Input: dimensioned drawing with shaded views. Units: mm. Origin: part minimum x, y, z. Give positions to 0.01 mm unless a question says otherwise; leave off trailing zeros. Write each loop counter-clockwise with the first axis right and the second up, starting at its lowest first coordinate (ties: lowest second). Pieces come first, ordered by that corner, then holes.
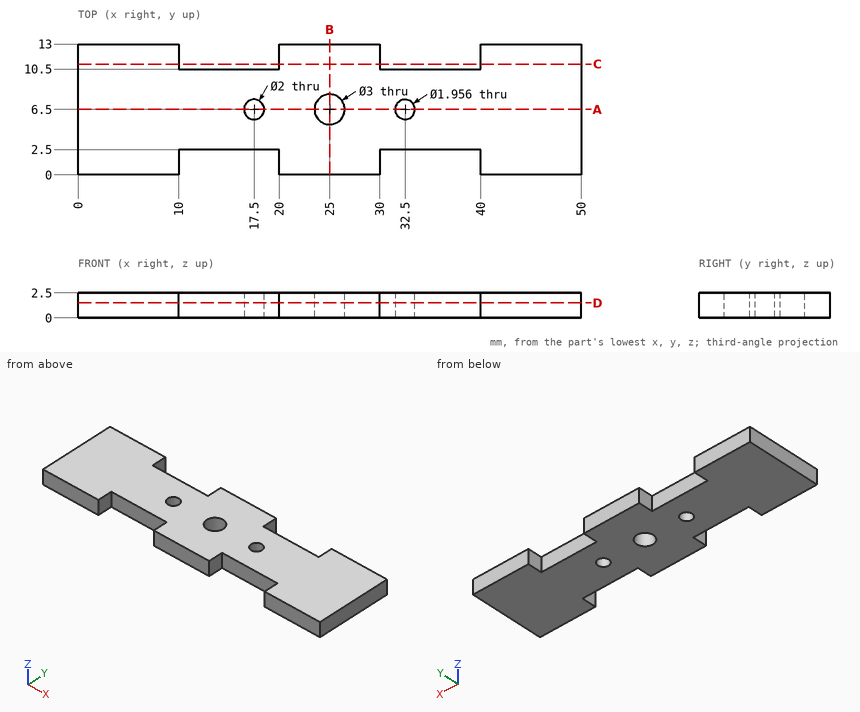
1. Cut plane B-B, the plane x = 25. Return the cut outline in (y, z), then the cut area to 3 significant figures.
2. Line query: L1, parallel to X at y = 1.5, z = 1.95; L2, parallel to Y at x = 17.5, z = 1.7; L3, parallel to X at y = 7, z = 1.45 (1 decimal). Output: solid intervals per line, ascending.
3. Cut plane C-C, the plane y = 11. Return the cut outline in (x, z).
4. Cut plane A-A, the plane y = 6.5. Return the cut outline in (x, z), then the cut area to 3 significant figures.
5. Contact query for flat-ended pins moving along their axis: P1, Ø1.2, axis at x = 13.5, z = 1.5, coming from the -Y side; P2, Ø1.2, axis at x = 15, z = 1.5, coming from the +Y side. Output: stop coordinate, or through.
6. Cut plane D-D, the plane z = 1.5. Return the cut outline in (x, y) (1 decimal), then the cut area to 3 significant figures.
Response values:
1. outline: (0, 0) - (5, 0) - (5, 2.5) - (0, 2.5) - close; (8, 0) - (13, 0) - (13, 2.5) - (8, 2.5) - close
1. area: 25.0 mm2
2. L1: x = 0 to 10, 20 to 30, 40 to 50
2. L2: y = 2.5 to 5.5, 7.5 to 10.5
2. L3: x = 0 to 16.6, 18.4 to 23.6, 26.4 to 31.7, 33.3 to 50
3. outline: (0, 0) - (10, 0) - (10, 2.5) - (0, 2.5) - close; (20, 0) - (30, 0) - (30, 2.5) - (20, 2.5) - close; (40, 0) - (50, 0) - (50, 2.5) - (40, 2.5) - close
4. outline: (0, 0) - (16.5, 0) - (16.5, 2.5) - (0, 2.5) - close; (18.5, 0) - (23.5, 0) - (23.5, 2.5) - (18.5, 2.5) - close; (26.5, 0) - (31.52, 0) - (31.52, 2.5) - (26.5, 2.5) - close; (33.48, 0) - (50, 0) - (50, 2.5) - (33.48, 2.5) - close
4. area: 108 mm2
5. P1: stops at y = 2.5
5. P2: stops at y = 10.5
6. outline: (0, 0) - (10, 0) - (10, 2.5) - (20, 2.5) - (20, 0) - (30, 0) - (30, 2.5) - (40, 2.5) - (40, 0) - (50, 0) - (50, 13) - (40, 13) - (40, 10.5) - (30, 10.5) - (30, 13) - (20, 13) - (20, 10.5) - (10, 10.5) - (10, 13) - (0, 13) - close; hole circle Ø2 at (17.5, 6.5); hole circle Ø3 at (25, 6.5); hole circle Ø2 at (32.5, 6.5)
6. area: 537 mm2
